```python
from build123d import *

# Parameters (mm, degrees)
SKETCH1_W               = 55
SKETCH1_H               = 55
SKETCH1_R               = 12.7
BOSS_EXTRUDE1_DEPTH     = 10.7
CUT_EXTRUDE1_DEPTH      = 41.335964102
CUT_EXTRUDE1_DEPTH_BACK = 41.335964102
SKETCH2_R               = 2
CHAMFER1_SIZE           = 0.25


with BuildPart() as part:
    # Sketch1 → Boss-Extrude1 (new body)
    with BuildSketch(Plane.XY):
        Rectangle(SKETCH1_W, SKETCH1_H)
        Circle(SKETCH1_R, mode=Mode.SUBTRACT)
    extrude(amount=BOSS_EXTRUDE1_DEPTH)

    # Sketch2 → Cut-Extrude1 (cut, two sides: drawn at the far end of the back side and taken through both)
    with BuildSketch(Plane(origin=(0, 0, 0), x_dir=(1, 0, 0), z_dir=(0, 1, 0)).offset(-CUT_EXTRUDE1_DEPTH_BACK)):
        with Locations(Location((0, -3.8, 0), (0, 0, 270))):
            Circle(SKETCH2_R)
    extrude(amount=CUT_EXTRUDE1_DEPTH + CUT_EXTRUDE1_DEPTH_BACK, mode=Mode.SUBTRACT)

    # Chamfer1
    chamfer1_edges = [part.edges().sort_by_distance(p)[0] for p in [
        (-12.7, 0, 0),
        (-12.7, 0, 10.7),
        (-27.5, 0, 10.7),
        (0, -27.5, 10.7),
        (27.5, 0, 10.7),
        (0, -27.5, 0),
        (-27.5, 0, 0),
        (0, 27.5, 0),
        (27.5, 0, 0),
        (0, 27.5, 10.7),
    ]]
    chamfer(chamfer1_edges, length=CHAMFER1_SIZE)


solid = part.part
```
The model under review builds one solid part; all positions refer to its coordinate system, in mm. Give positions to 0.01 mm unless a question says otherwise; leave off trailing zeros. Write each loop counter-clockwise with the first axis right and the second up, starting at its lowest first coordinate (ties: lowest second). Pieces come first, ordered by that corner, then holes. Notation, with made-up numbers: M -12,58.5 L 9,58.5 A11 cw 9,69.5 Z; hole C 87.25,4.25 d5. An arc over 180 degrees is marked long. Write each question's results on one line, items separated by ' | '. Start each with the question number.
1. We need section B-B (y = 0). Write out the cut boundary in (x, z), and give its area (3 significant figures).
2. Mouldability with a two-part tool opening along X and no side actions: class faces 1 (the flat face through (-27.5, 0, 5)), 2 (the flat face through (27.5, 0, 5)), 3 (the cylindrical face through (-2.75, -12.4, 5.28)), 4 (the flat face through (0, 27.5, 6)) as released by +X, released by -X, zero draft, split by the parting line, or undercut.
3. We need section D-D (y = 19). Write out the cut boundary in (x, z), and give its area (3 significant figures).
4. We need section C-C (z = 3.8). Write out the cut boundary in (x, y).
5. For probe 1 along Z at (x, y) = (0, -15.25); probe 2 along X at (y, z) = (-19.5, 3.8); probe 3 along Y at (x, z) = (-0.5, 0.75), list the stretches that pass through material, from the lowest coordinate up. Write a range as [from, to].
6. We need section A-A (x = 0). Write out the cut boundary in (y, z).
7. Insertion check: pin 1 Ø5 at (x, z) = (0, 3.8) entering from +Y; pin 2 Ø20.5 at (x, y) = (0, 0) entering from +Z. Each pin has a flat end and moves straight along its axis. Give the tip position at first contact, or say it passes through.
Results found:
1) outline: M -27.5,0.25 L -27.25,0 L -12.95,0 L -12.7,0.25 L -12.7,10.45 L -12.95,10.7 L -27.25,10.7 L -27.5,10.45 Z; M 12.7,0.25 L 12.95,0 L 27.25,0 L 27.5,0.25 L 27.5,10.45 L 27.25,10.7 L 12.95,10.7 L 12.7,10.45 Z | area: 316 mm^2
2) face 1: released by -X | face 2: released by +X | face 3: undercut | face 4: zero draft
3) outline: M -27.5,0.25 L -27.25,0 L 27.25,0 L 27.5,0.25 L 27.5,10.45 L 27.25,10.7 L -27.25,10.7 L -27.5,10.45 Z; hole C 0,3.8 d4 | area: 576 mm^2
4) outline: M -27.5,-27.5 L -2,-27.5 L -2,-12.54 A12.7 cw -2,12.54 L -2,27.5 L -27.5,27.5 Z; M 2,-27.5 L 27.5,-27.5 L 27.5,27.5 L 2,27.5 L 2,12.54 A12.7 cw 2,-12.54 Z
5) probe 1: z = [0, 1.8], [5.8, 10.7] | probe 2: x = [-27.5, -2], [2, 27.5] | probe 3: y = [-27.5, -12.69], [12.69, 27.5]
6) outline: M -27.5,0.25 L -27.25,0 L -12.95,0 L -12.7,0.25 L -12.7,1.8 L -27.5,1.8 Z; M -27.5,5.8 L -12.7,5.8 L -12.7,10.45 L -12.95,10.7 L -27.25,10.7 L -27.5,10.45 Z; M 12.7,0.25 L 12.95,0 L 27.25,0 L 27.5,0.25 L 27.5,1.8 L 12.7,1.8 Z; M 12.7,5.8 L 27.5,5.8 L 27.5,10.45 L 27.25,10.7 L 12.95,10.7 L 12.7,10.45 Z
7) pin 1: stops at y = 27.5 | pin 2: passes through
